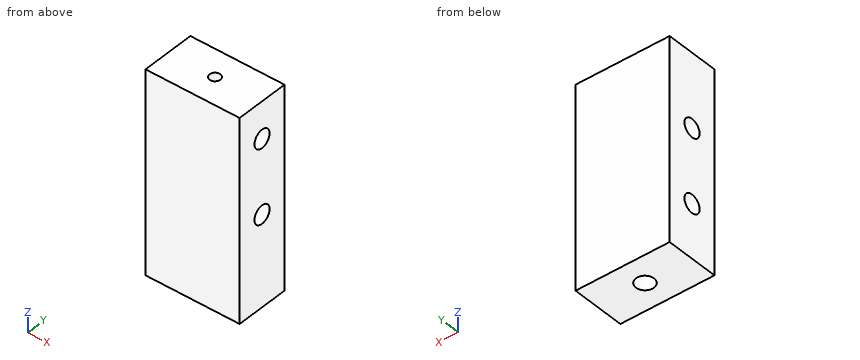
```python
from build123d import *

# Parameters (mm, degrees)
SKETCH1_W           = 44.45
SKETCH1_H           = 25.4
BOSS_EXTRUDE1_DEPTH = 95.25
SKETCH2_R           = 4.28
CUT_EXTRUDE1_DEPTH  = 14.224
SKETCH3_R           = 4.28
CUT_EXTRUDE2_DEPTH  = 14.224
SKETCH5_R           = 4.2799
CUT_EXTRUDE4_DEPTH  = 14.224
SKETCH6_R           = 2.54
CUT_EXTRUDE5_DEPTH  = 86.36
CUT_EXTRUDE6_REACH  = 32.226
SKETCH7_R           = 2.54
CUT_EXTRUDE7_REACH  = 32.226
SKETCH8_R           = 2.54


with BuildPart() as part:
    # Sketch1 → Boss-Extrude1 (new body)
    with BuildSketch(Plane.XY):
        with Locations((22.225, 12.7)):
            Rectangle(SKETCH1_W, SKETCH1_H)
    extrude(amount=BOSS_EXTRUDE1_DEPTH)

    # Sketch2 → Cut-Extrude1 (cut)
    with BuildSketch(Plane.ZY):
        with Locations((25.4, 12.7)):
            Circle(SKETCH2_R)
        with Locations((60.4, 12.7)):
            Circle(SKETCH2_R)
    extrude(amount=-CUT_EXTRUDE1_DEPTH, mode=Mode.SUBTRACT)

    # Sketch3 → Cut-Extrude2 (cut)
    with BuildSketch(Plane(origin=(44.45, 0, 0), x_dir=(0, 0, -1), z_dir=(1, 0, 0))):
        with Locations((-77.9, 12.7)):
            Circle(SKETCH3_R)
        with Locations((-42.9, 12.7)):
            Circle(SKETCH3_R)
    extrude(amount=-CUT_EXTRUDE2_DEPTH, mode=Mode.SUBTRACT)

    # Sketch5 → Cut-Extrude4 (cut)
    with BuildSketch(Plane(origin=(0, 0, 0), x_dir=(-1, 0, 0), z_dir=(0, 0, -1))):
        with Locations((-22.225, 12.7)):
            Circle(SKETCH5_R)
    extrude(amount=-CUT_EXTRUDE4_DEPTH, mode=Mode.SUBTRACT)

    # Sketch6 → Cut-Extrude5 (cut)
    with BuildSketch(Plane(origin=(0, 0, 14.224), x_dir=(-1, 0, 0), z_dir=(0, 0, -1))):
        with Locations((-22.225, 12.7)):
            Circle(SKETCH6_R)
    extrude(amount=-CUT_EXTRUDE5_DEPTH, mode=Mode.SUBTRACT)

    # Sketch7 → Cut-Extrude6 (cut, up to next)
    with BuildSketch(Plane(origin=(30.226, 0, 0), x_dir=(0, 0, -1), z_dir=(1, 0, 0)), mode=Mode.PRIVATE) as cut_extrude6_sk1:
        with Locations((-42.9, 12.7)):
            Circle(SKETCH7_R)
    cut_extrude6_tool1 = extrude(cut_extrude6_sk1.sketch, amount=-CUT_EXTRUDE6_REACH, mode=Mode.PRIVATE) & part.part
    add(cut_extrude6_tool1.solids().sort_by_distance((30.226, 12.7, 42.9))[0], mode=Mode.SUBTRACT)
    # Sketch7 → Cut-Extrude6 (cut, up to next)
    with BuildSketch(Plane(origin=(30.226, 0, 0), x_dir=(0, 0, -1), z_dir=(1, 0, 0)), mode=Mode.PRIVATE) as cut_extrude6_sk2:
        with Locations((-77.9, 12.7)):
            Circle(SKETCH7_R)
    cut_extrude6_tool2 = extrude(cut_extrude6_sk2.sketch, amount=-CUT_EXTRUDE6_REACH, mode=Mode.PRIVATE) & part.part
    add(cut_extrude6_tool2.solids().sort_by_distance((30.226, 12.7, 77.9))[0], mode=Mode.SUBTRACT)

    # Sketch8 → Cut-Extrude7 (cut, up to next)
    with BuildSketch(Plane.ZY.offset(-14.224), mode=Mode.PRIVATE) as cut_extrude7_sk1:
        with Locations((25.4, 12.7)):
            Circle(SKETCH8_R)
    cut_extrude7_tool1 = extrude(cut_extrude7_sk1.sketch, amount=-CUT_EXTRUDE7_REACH, mode=Mode.PRIVATE) & part.part
    add(cut_extrude7_tool1.solids().sort_by_distance((14.224, 12.7, 25.4))[0], mode=Mode.SUBTRACT)
    # Sketch8 → Cut-Extrude7 (cut, up to next)
    with BuildSketch(Plane.ZY.offset(-14.224), mode=Mode.PRIVATE) as cut_extrude7_sk2:
        with Locations((60.4, 12.7)):
            Circle(SKETCH8_R)
    cut_extrude7_tool2 = extrude(cut_extrude7_sk2.sketch, amount=-CUT_EXTRUDE7_REACH, mode=Mode.PRIVATE) & part.part
    add(cut_extrude7_tool2.solids().sort_by_distance((14.224, 12.7, 60.4))[0], mode=Mode.SUBTRACT)


solid = part.part
```
Design review of the part built by this model. Coordinates are the model's own, in mm. Coordinates: 2 decimals unless noted, no trailing zeros. Loops run counter-clockwise (first coordinate to the right, second up) from the corner with the lowest first, then second, coordinate; pieces in that order, holes last.
Q1. For pin 1 (2.5 mm diameter, centred on y = 11, z = 26, fed in from -X); pin 2 (7.5 mm diameter, centred on x = 22.225, y = 12.7, fed in from -Z), all flat-tipped, find the tip position at first contact; note any pin that passes through.
Reported:
pin 1: stops at x = 14.22
pin 2: stops at z = 14.22
Q2. We need section A-A on z = 42.9. State the section outline as (x, y) points (3 decimals), and give its area (3 significant figures).
Reported:
outline: (0, 0) - (44.45, 0) - (44.45, 8.42) - (30.226, 8.42) - (30.226, 10.16) - (22.225, 10.16) arc R2.54 cw to (22.225, 15.24) - (30.226, 15.24) - (30.226, 16.98) - (44.45, 16.98) - (44.45, 25.4) - (0, 25.4) - close
area: 956 mm2
Q3. We need section C-C on z = 67.5. State the section outline as (x, y) points (3 decimals), and give its area (3 significant figures).
Reported:
outline: (0, 0) - (44.45, 0) - (44.45, 25.4) - (0, 25.4) - close; hole circle Ø5.08 at (22.225, 12.7)
area: 1,110 mm2
Q4. To check wall thickness, follow line 1 (Y direction, x = 10, z = 60); line 2 (Z direction, x = 19.5, y = 12.7); line 3 (Y direction, x = 17, z = 25.4). State the ranges of each line that lie inside material, in increasing order.
Reported:
line 1: y = 0 to 8.44, 16.96 to 25.4
line 2: z = 14.22 to 22.86, 27.94 to 57.86, 62.94 to 95.25
line 3: y = 0 to 10.16, 15.24 to 25.4
Q5. We need section B-B on x = 31.5. State the section outline as (y, z) points, and give its area (3 significant figures).
Reported:
outline: (0, 0) - (25.4, 0) - (25.4, 95.25) - (0, 95.25) - close; hole circle Ø8.56 at (12.7, 42.9); hole circle Ø8.56 at (12.7, 77.9)
area: 2,300 mm2
Q6. We need section D-D on y = 12.7. State how many separate pieces and enclosed holes the cut face has, and give its area (3 significant figures).
Reported:
separate pieces: 6
enclosed holes: 0
area: 3,100 mm2
